```python
from build123d import *

# Parameters (mm, degrees)
SKETCH1_W           = 145
SKETCH1_H           = 55
BOSS_EXTRUDE1_DEPTH = 3.175
SKETCH4_R           = 0.75
SKETCH4_R_2         = 19.05
CUT_EXTRUDE1_DEPTH  = 156.113122027


with BuildPart() as part:
    # Sketch1 → Boss-Extrude1 (new body)
    with BuildSketch(Plane(origin=(0, 0, 0), x_dir=(1, 0, 0), z_dir=(0, 1, 0))):
        with Locations((72.5, 27.5)):
            Rectangle(SKETCH1_W, SKETCH1_H)
    extrude(amount=BOSS_EXTRUDE1_DEPTH)

    # Sketch4 → Cut-Extrude1 (cut, through all)
    with BuildSketch(Plane.XZ):
        with Locations(Location((10.25, -11.5, 0), (0, 0, 270))):
            Circle(SKETCH4_R)
        with Locations(Location((10.25, -43.5, 0), (0, 0, 270))):
            Circle(SKETCH4_R)
        with Locations(Location((42.25, -43.5, 0), (0, 0, 270))):
            Circle(SKETCH4_R)
        with Locations(Location((26.25, -27.5, 0), (0, 0, 270))):
            Circle(SKETCH4_R_2)
        with Locations(Location((42.25, -11.5, 0), (0, 0, 270))):
            Circle(SKETCH4_R)
        with Locations(Location((56.5, -11.5, 0), (0, 0, 270))):
            Circle(SKETCH4_R)
        with Locations(Location((56.5, -43.5, 0), (0, 0, 270))):
            Circle(SKETCH4_R)
        with Locations(Location((88.5, -43.5, 0), (0, 0, 270))):
            Circle(SKETCH4_R)
        with Locations(Location((88.5, -11.5, 0), (0, 0, 270))):
            Circle(SKETCH4_R)
        with Locations(Location((72.5, -27.5, 0), (0, 0, 270))):
            Circle(SKETCH4_R_2)
        with Locations(Location((102.75, -11.5, 0), (0, 0, 270))):
            Circle(SKETCH4_R)
        with Locations(Location((102.75, -43.5, 0), (0, 0, 270))):
            Circle(SKETCH4_R)
        with Locations(Location((134.75, -43.5, 0), (0, 0, 270))):
            Circle(SKETCH4_R)
        with Locations(Location((134.75, -11.5, 0), (0, 0, 270))):
            Circle(SKETCH4_R)
        with Locations(Location((118.75, -27.5, 0), (0, 0, 270))):
            Circle(SKETCH4_R_2)
        with Locations(Location((4.750000369, -48.50000744, 0), (0, 0, 270))):
            Circle(SKETCH4_R)
        with Locations(Location((4.749998796, -5.00000808, 0), (0, 0, 270))):
            Circle(SKETCH4_R)
        with Locations(Location((140.249999576, -5.00000318, 0), (0, 0, 270))):
            Circle(SKETCH4_R)
        with Locations(Location((140.250001149, -48.50000254, 0), (0, 0, 270))):
            Circle(SKETCH4_R)
        with BuildLine():
            Line((113.775, -51.825), (113.775, -55))
            Line((113.775, -55), (31.225, -55))
            Line((31.225, -55), (31.225, -51.825))
            ThreePointArc((31.225, -51.825), (32.15493597, -49.57993597), (34.4, -48.65))
            Line((34.4, -48.65), (110.6, -48.65))
            ThreePointArc((110.6, -48.65), (112.84506403, -49.57993597), (113.775, -51.825))
        make_face()
    extrude(amount=-CUT_EXTRUDE1_DEPTH, mode=Mode.SUBTRACT)


solid = part.part
```
The listing builds one solid part. Answer for the finished solid, in the listing's coordinates (mm). A direction names the side the tool comes from. Give positions to 0.01 mm unless a question says otherwise; leave off trailing zeros. Loops run counter-clockwise (first coordinate to the right, second up) from the corner with the lowest first, then second, coordinate; pieces in that order, holes last. Notation, with made-up numbers: M -23.75,-16 L 2.25,-16 A21 ccw 2.25,6 Z; hole C 87,-20.75 d1. An arc over 180 degrees is marked long. One line per item, written item: value.
1. Section C-C on z = -26.5 is taken. Determine the outline of the cut face in (x, y) (3 decimals).
Found:
outline: M 0,0 L 7.226,0 L 7.226,3.175 L 0,3.175 Z; M 45.274,0 L 53.476,0 L 53.476,3.175 L 45.274,3.175 Z; M 91.524,0 L 99.726,0 L 99.726,3.175 L 91.524,3.175 Z; M 137.774,0 L 145,0 L 145,3.175 L 137.774,3.175 Z
2. For faces 4 (the face through (129, 2, -55)), 5 (the face through (31.225, 2, -53)), determine the directions among +Z, -Z, +X, -X, +Y, -Y from which every point of the face is accessible in a straight line to the end or side of a thin tool.
Found:
face 4: -Z, +X, -X, +Y, -Y
face 5: -Z, +Y, -Y
3. Section A-A on x = 72.5 is taken. Determine the outline of the cut face in (y, z) (3 decimals).
Found:
outline: M 0,-48.65 L 3.175,-48.65 L 3.175,-46.55 L 0,-46.55 Z; M 0,-8.45 L 3.175,-8.45 L 3.175,0 L 0,0 Z
4. Find the intervals of material crossed by probe 1 along X at (y, z) = (0.85, -27.5); probe 2 along X at (y, z) = (2.5, -12.5); probe 3 along Z at (x, y) = (56.5, 2.55), in increasing order.
Found:
probe 1: 0 to 7.2, 45.3 to 53.45, 91.55 to 99.7, 137.8 to 145
probe 2: 0 to 14.51, 37.99 to 60.76, 84.24 to 107.01, 130.49 to 145
probe 3: -48.65 to -44.25, -42.75 to -37.84, -17.16 to -12.25, -10.75 to 0
5. Section D-D on x = 16.5 is taken. Determine the outline of the cut face in (y, z) (3 decimals), plus the area to 3 significant figures.
Found:
outline: M 0,-55 L 3.175,-55 L 3.175,-43.866 L 0,-43.866 Z; M 0,-11.134 L 3.175,-11.134 L 3.175,0 L 0,0 Z
area: 70.7 mm^2
6. Section B-B on y = 1.8 is taken. State how many separate pieces and enclosed holes the cut face has, plus the area to 3 significant figures.
Found:
separate pieces: 1
enclosed holes: 19
area: 4,010 mm^2
7. For a pull along X with two mould halves and no side action, classify faces 1 (the face through (113.775, 2, -53)), 2 (the face through (71, 2, 0)), 3 (the face through (0, 2, -27)) as pulls with the +X half, pulls with the -X half, needs draft (parallel to the pull), parting line crosses it, or undercut.
Found:
face 1: undercut
face 2: needs draft
face 3: pulls with the -X half
